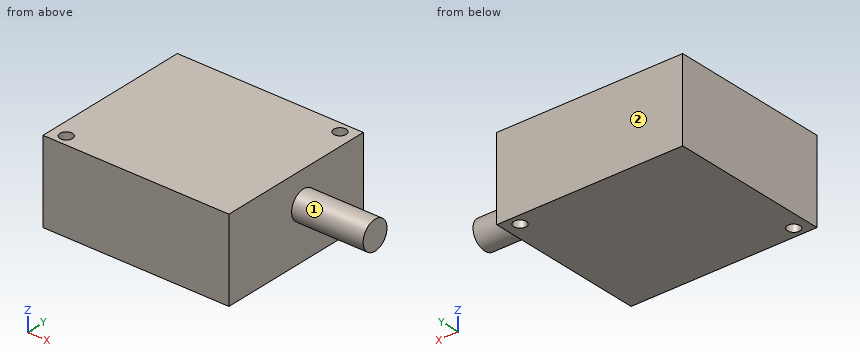
```python
from build123d import *

# Parameters (mm, degrees)
SKETCH_W     = 52
SKETCH_H     = 45
SKETCH_R     = 1.75
PAD_DEPTH    = 23
SKETCH001_R  = 4
PAD001_DEPTH = 20


with BuildPart() as part:
    # Sketch → Pad (new body)
    with BuildSketch(Plane.XY):
        Rectangle(SKETCH_W, SKETCH_H)
        with Locations((-22, -19.5)):
            Circle(SKETCH_R, mode=Mode.SUBTRACT)
        with Locations((22, 19.5)):
            Circle(SKETCH_R, mode=Mode.SUBTRACT)
    extrude(amount=PAD_DEPTH)

    # Sketch001 (on Face2 of Pad) → Pad001 (join)
    with BuildSketch(Plane.YZ.offset(26)):
        with Locations((2.5, 14)):
            Circle(SKETCH001_R)
    extrude(amount=PAD001_DEPTH)


solid = part.part
```
The model under review builds one solid part; all positions refer to its coordinate system, in mm. Face numbers are marked on the shaded views. A direction names the side the tool comes from. Round coordinates to 2 decimals unless told otherwise and drop trailing zeros. Write each loop counter-clockwise with the first axis right and the second up, starting at its lowest first coordinate (ties: lowest second). Pieces come first, ordered by that corner, then holes.
(1) We need section D-D on y = 0.5. Give the boundary of the cut face in (x, z), and give its area (3 significant figures).
(2) We need section A-A on y = 19.5. Give the boundary of the cut face in (x, z), and give its area (3 significant figures).
(3) Insertion check: pin 1 (1.5 mm diameter, centred on x = 35, z = 10, fed in from -Y); pin 2 (8 mm diameter, centred on y = 15.5, z = 9.5, fed in from +X). Each pin has a flat end and moves straight along its axis. Give the tip position at first contact, or say it passes through.
(4) We need section C-C on z = 5.25. Give the boundary of the cut face in (x, y), and give its area (3 significant figures).
(5) Wall thickness on L1, parallel to Y at x = -22, z = 10.75; L2, parallel to Y at x = 22, z = 7.5; L3, parallel to X at y = -17.5, z = 11.25: over which ranges is each line inside the solid? List them lowest first.
(6) We need section B-B on x = -22. Give the boundary of the cut face in (y, z).
(7) Machinability: for the marked faces 1 and 2, which of the approach directions +Z, -Z, +X, -X, +Y, -Y give a long, thin tool a straight path to every point of the face, cutting with its end or side? Answer none if there is none.
Findings below:
1. outline: (-26, 0) - (26, 0) - (26, 10.54) - (46, 10.54) - (46, 17.46) - (26, 17.46) - (26, 23) - (-26, 23) - close
1. area: 1,330 mm2
2. outline: (-26, 0) - (20.25, 0) - (20.25, 23) - (-26, 23) - close; (23.75, 0) - (26, 0) - (26, 23) - (23.75, 23) - close
2. area: 1,120 mm2
3. pin 1: stops at y = 0.17
3. pin 2: stops at x = 26
4. outline: (-26, -22.5) - (26, -22.5) - (26, 22.5) - (-26, 22.5) - close; hole circle Ø3.5 at (-22, -19.5); hole circle Ø3.5 at (22, 19.5)
4. area: 2,320 mm2
5. L1: y = -22.5 to -21.25, -17.75 to 22.5
5. L2: y = -22.5 to 17.75, 21.25 to 22.5
5. L3: x = -26 to 26
6. outline: (-22.5, 0) - (-21.25, 0) - (-21.25, 23) - (-22.5, 23) - close; (-17.75, 0) - (22.5, 0) - (22.5, 23) - (-17.75, 23) - close
7. face 1: +X
7. face 2: +Z, -Z, +X, -X, +Y
